```python
from build123d import *

# Parameters (mm, degrees)
BASPROSKE_W         = 5.5
BASPROSKE_H         = 13.5
TOOTHCUT_DEPTH      = 20.868316486
TEETHCUTS_COUNT     = 25
TEETHCUTS_ANGLE     = 345.6
BORSKE_R            = 7
BORE_DEPTH          = 50.0000508
EXTRUDE_START       = -5.5
SKETCH_1_R          = 7
EXTRUDE_1_DEPTH     = 5.5
SKETCH_2_R          = 1.6
CUT_EXTRUDE_1_DEPTH = 20.860181149


with BuildPart() as part:
    # BasProSke → Base-Revolve (revolve)
    with BuildSketch(Plane(origin=(0, 0, 0), x_dir=(1, 0, 0), z_dir=(0, 1, 0)), mode=Mode.PRIVATE) as base_revolve_sk:
        with Locations((2.75, 6.75)):
            Rectangle(BASPROSKE_W, BASPROSKE_H)
    revolve(base_revolve_sk.sketch.rotate(Axis((-10, 0, 0), (1, 0, 0)), 180), axis=Axis((-10, 0, 0), (1, 0, 0)))

    # TooCutSke → ToothCut (cut, through all)
    with BuildSketch(Plane(origin=(0, 0, 0), x_dir=(0, 0, -1), z_dir=(1, 0, 0))):
        with BuildLine():
            ThreePointArc((0.480087995, 11.238750665), (0, 11.249), (-0.480087995, 11.238750665))
            ThreePointArc((-0.480087995, 11.238750665), (-0.821124963, 12.40220054), (-1.432168974, 13.449361962))
            ThreePointArc((-1.432168974, 13.449361962), (0, 13.5254), (1.432168974, 13.449361962))
            ThreePointArc((1.432168974, 13.449361962), (0.821124963, 12.40220054), (0.480087995, 11.238750665))
        make_face()
    toothcut = extrude(amount=TOOTHCUT_DEPTH, mode=Mode.SUBTRACT)

    # TeethCuts: ToothCut ×25 about axis
    teethcuts_axis = Axis((-10, 0, 0), (1, 0, 0))
    for i in range(1, TEETHCUTS_COUNT):
        add(toothcut.rotate(teethcuts_axis, i * TEETHCUTS_ANGLE / (TEETHCUTS_COUNT - 1)), mode=Mode.SUBTRACT)

    # BorSke → Bore (cut, symmetric)
    with BuildSketch(Plane(origin=(0, 0, 0), x_dir=(0, 0, -1), z_dir=(1, 0, 0))):
        with Locations(Location((0, 0, 0), (0, 0, 180))):
            Circle(BORSKE_R)
    extrude(amount=BORE_DEPTH, both=True, mode=Mode.SUBTRACT)

    # ｽｹｯﾁ1 → ﾎﾞｽ - 押し出し1 (add)
    with BuildSketch(Plane.ZY.offset(EXTRUDE_START)):
        Circle(SKETCH_1_R)
    extrude(amount=EXTRUDE_1_DEPTH)

    # ｽｹｯﾁ2 → ｶｯﾄ - 押し出し1 (cut, through all)
    with BuildSketch(Plane(origin=(5.5, 0, 0), x_dir=(0, 0, -1), z_dir=(1, 0, 0))):
        with Locations((0, 7)):
            Circle(SKETCH_2_R)
        with Locations((7, 0)):
            Circle(SKETCH_2_R)
        with Locations((0, -7)):
            Circle(SKETCH_2_R)
        with Locations((-7, 0)):
            Circle(SKETCH_2_R)
    extrude(amount=-CUT_EXTRUDE_1_DEPTH, mode=Mode.SUBTRACT)


solid = part.part
```
For this review, take the finished solid that the model builds, in its own axes (mm). A direction names the side the tool comes from. Coordinates: 2 decimals unless noted, no trailing zeros. Loops run counter-clockwise (first coordinate to the right, second up) from the corner with the lowest first, then second, coordinate; pieces in that order, holes last.
1. Insertion check: P1, Ø1.5, axis at x = 2.5, z = -2.5, coming from the -Y side. The pin has a flat end and moves straight along its axis. Give the tip position at first contact, or say it passes through.
2. Add section B-B, the plane x = 0.4. Count the separate pieces of the cut face and the enclosed holes in it, then the cut area to 3 significant figures.
3. Add section C-C, the plane z = -2.75. Give the boundary of the cut face in (x, y).
4. For faces 4 (the cylindrical face through (2.71, -11.16, 1.42)), 5 (the cylindrical face through (2.71, 12.4, -0.82)), 6 (the cylindrical face through (2.712, 0.7, -11.227)), 7 (the cylindrical face through (2.71, -3.11, 12)), 8 (the cylindrical face through (2.712, 11.266, 5.255)), list the 3-axis set-ups (+Z, -Z, +X, -X, +Y, -Y) from which the entire face can be reached by the end or side of a thin tool; tool diameter is ignored.
5. Add section A-A, the plane y = 7. Give the boundary of the cut face in (x, z), then the cut area to 3 significant figures.
6. Mouldability with a two-part tool opening along Y and no side actions: class faces 1 (the cylindrical face through (2.712, 10.453, 6.669)), 2 (the cylindrical face through (2.712, 6.022, -9.501)), 3 (the cylindrical face through (2.712, -9.552, 7.956)) as +Y half, -Y half, draft (parallel to the pull), parting line (faces both ways), or undercut.
7. For line 1 (Y direction, x = 2.25, z = 0); line 2 (Z direction, x = 2.65, y = 11.75); line 3 (Y direction, x = 2.65, z = -1.25), list the stretches that pass through material, from the lowest coordinate up.
Result:
1. P1: stops at y = -13.14
2. separate pieces: 1
2. enclosed holes: 4
2. area: 445 mm2
3. outline: (0, -12.76) - (5.5, -12.76) - (5.5, 10.91) - (0, 10.91) - close
4. face 4: +X, -X, -Y
4. face 5: +X, -X, +Y
4. face 6: -Z, +X, -X
4. face 7: +Z, +X, -X
4. face 8: +X, -X
5. outline: (0, -9.78) - (5.5, -9.78) - (5.5, -1.6) - (0, -1.6) - close; (0, 1.6) - (5.5, 1.6) - (5.5, 9.78) - (0, 9.78) - close
5. area: 90.0 mm2
6. face 1: +Y half
6. face 2: undercut
6. face 3: -Y half
7. line 1: y = -13.5 to -8.6, -5.4 to 5.4, 8.6 to 11.25
7. line 2: z = -5.28 to -3.84, -2.34 to -0.59, 0.59 to 2.34, 3.84 to 5.28
7. line 3: y = -11.18 to -8, -6 to 6, 8 to 13.19
